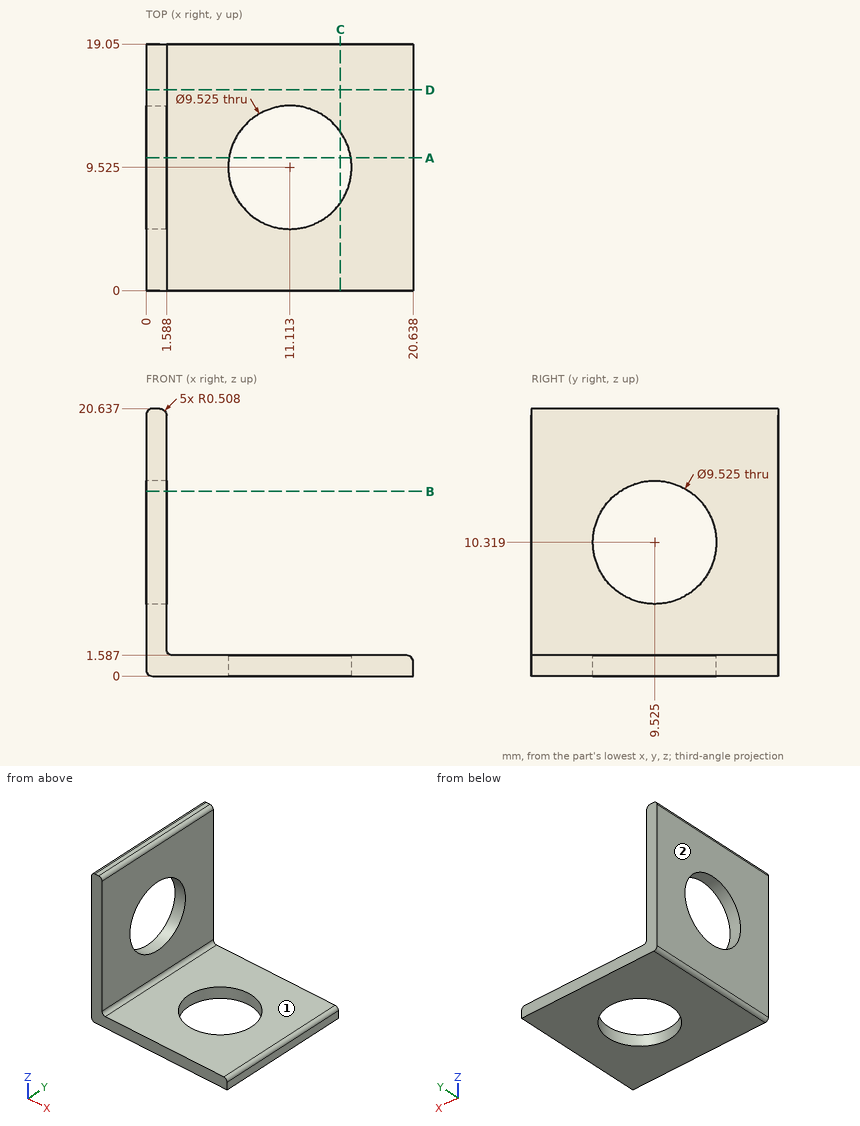
The figure shows three views and two pictorial views of one solid part (mm, origin at its lowest corner). Answer the questions. A direction names the side the tool comes from. Coordinates: 2 decimals unless noted, no trailing zeros. Loops run counter-clockwise (first coordinate to the right, second up) from the corner with the lowest first, then second, coordinate; pieces in that order, holes last. Notation, with made-up numbers: (-30.75, 55) - (-2.75, 55) arc R14 cw to (-2.75, 73) - close; hole circle Ø1 at (8, 19). An arc over 180 degrees is marked (long way). Answer in a Markdown table with one row per item.
Q1. Find section C-C on x = 15. Write down the section's boundary in (y, z).
Here are the results:
| item | result |
|---|---|
| outline | (0, 0) - (6.77, 0) - (6.77, 1.59) - (0, 1.59) - close; (12.28, 0) - (19.05, 0) - (19.05, 1.59) - (12.28, 1.59) - close |
Q2. For the marked faces 1 and 2, determine the directions among +Z, -Z, +X, -X, +Y, -Y from which every point of the face is accessible in a straight line to the end or side of a thin tool.
Here are the results:
| item | result |
|---|---|
| face 1 | +Z, +X, +Y, -Y |
| face 2 | +Z, -Z, -X, +Y, -Y |
Q3. Find section D-D on y = 15.5. Write down the section's boundary in (x, z) (1 decimal).
Here are the results:
| item | result |
|---|---|
| outline | (0, 0.5) arc R0.5 ccw to (0.5, 0) - (20.6, 0) - (20.6, 1.1) arc R0.5 ccw to (20.1, 1.6) - (2.1, 1.6) arc R0.5 cw to (1.6, 2.1) - (1.6, 20.1) arc R0.5 ccw to (1.1, 20.6) - (0.5, 20.6) arc R0.5 ccw to (0, 20.1) - close |
Q4. Given P1, Ø3, axis at y = 14.5, z = 14.5, coming from the +X side; P2, Ø1.5, axis at x = 3, z = 14, coming from the +Y side, each flat-ended and moving along its own axis, determine where each tip first touches the part or whether it passes through.
Here are the results:
| item | result |
|---|---|
| P1 | stops at x = 1.59 |
| P2 | passes through |
Q5. Find section A-A on y = 10.25. Write down the section's boundary in (x, z) (1 decimal).
Here are the results:
| item | result |
|---|---|
| outline | (0, 0.5) arc R0.5 ccw to (0.5, 0) - (6.4, 0) - (6.4, 1.6) - (2.1, 1.6) arc R0.5 cw to (1.6, 2.1) - (1.6, 5.6) - (0, 5.6) - close; (0, 15) - (1.6, 15) - (1.6, 20.1) arc R0.5 ccw to (1.1, 20.6) - (0.5, 20.6) arc R0.5 ccw to (0, 20.1) - close; (15.8, 0) - (20.6, 0) - (20.6, 1.1) arc R0.5 ccw to (20.1, 1.6) - (15.8, 1.6) - close |
Q6. Straight lines are drawn through the part: line 1 along X through (y, z) = (3.5, 9.5); line 2 along X through (y, z) = (14.25, 1.75) (1 decimal). For each, find the intervals that lie inside material, in ascending order. Write a range as [from, to].
Here are the results:
| item | result |
|---|---|
| line 1 | x = [0, 1.59] |
| line 2 | x = [0, 1.7] |
Q7. Find section B-B on z = 14.25. Write down the section's boundary in (x, y), plus the area to 3 significant figures.
Here are the results:
| item | result |
|---|---|
| outline | (0, 0) - (1.59, 0) - (1.59, 6.84) - (0, 6.84) - close; (0, 12.21) - (1.59, 12.21) - (1.59, 19.05) - (0, 19.05) - close |
| area | 21.7 mm^2 |
